from build123d import *

# Parameters (mm, degrees)
SKETCH_1_R               = 34.375
EXTRUDE_1_DEPTH          = 30
EXTRUDE_START            = -30
EXTRUDE_2_DEPTH          = 30
PATTERN_CIRCULAR_1_COUNT = 30
CUT_EXTRUDE_1_DEPTH      = 30


with BuildPart() as part:
    # 草图1 → 凸台-拉伸1 (new body)
    with BuildSketch(Plane.XY):
        Circle(SKETCH_1_R)
    extrude(amount=EXTRUDE_1_DEPTH)

    # 草图2 → 凸台-拉伸2 (add)
    with BuildSketch(Plane.XY.offset(30).offset(EXTRUDE_START)):
        with BuildLine():
            ThreePointArc((2.965504601, 39.889920813), (2.09343825, 39.94518139), (1.220372866, 39.981379292))
            ThreePointArc((1.220372866, 39.981379292), (-0.075113847, 37.287853424), (-0.712008739, 34.367625297))
            ThreePointArc((-0.712008739, 34.367625297), (1.799048496, 34.327890257), (4.300503339, 34.10493067))
            ThreePointArc((4.300503339, 34.10493067), (3.972344382, 37.075735127), (2.965504601, 39.889920813))
        make_face()
    extrude_2 = extrude(amount=EXTRUDE_2_DEPTH)

    # 阵列(圆周)1: 凸台-拉伸2 ×30 about axis
    pattern_circular_1_axis = Axis((0, 0, 0), (0, 0, 1))
    for i in range(1, PATTERN_CIRCULAR_1_COUNT):
        add(extrude_2.rotate(pattern_circular_1_axis, i * 360 / PATTERN_CIRCULAR_1_COUNT))

    # 草图3 → 切除-拉伸1 (cut)
    with BuildSketch(Plane.XY.offset(30)):
        with BuildLine():
            Line((-1.5, 14.924811557), (-1.5, 0))
            Line((-1.5, 0), (1.5, 0))
            Line((1.5, 0), (1.5, 14.924811557))
            ThreePointArc((1.5, 14.924811557), (0, 15), (-1.5, 14.924811557))
        make_face()
        with BuildLine():
            Line((1.5, 0), (-1.5, 0))
            Line((-1.5, 0), (-1.5, 14.924811557))
            ThreePointArc((-1.5, 14.924811557), (-10.062305899, -11.124297731), (15, 0))
            ThreePointArc((15, 0), (11.124297731, 10.062305899), (1.5, 14.924811557))
            Line((1.5, 14.924811557), (1.5, 0))
        make_face()
        with BuildLine():
            Line((-1.5, 17), (-1.5, 14.924811557))
            ThreePointArc((-1.5, 14.924811557), (0, 15), (1.5, 14.924811557))
            Line((1.5, 14.924811557), (1.5, 17))
            Line((1.5, 17), (-1.5, 17))
        make_face()
    extrude(amount=-CUT_EXTRUDE_1_DEPTH, mode=Mode.SUBTRACT)


solid = part.part
Could you check a few things on this model? Use its own coordinates, in mm. A direction names the side the tool comes from. Give positions to 0.01 mm unless a question says otherwise; leave off trailing zeros. Write each question's results on one line, items separated by ' | '. Start each with the question number.
Q1. I need wall thicknesses on probe 1 along X at (y, z) = (6, 15.75); probe 2 along Y at (x, z) = (10.5, 3.5); probe 3 along X at (y, z) = (24, 18). Which ranges of each line are inside material? Lowest first, please.
Q2. Which directions (+Z, -Z, +X, -X, +Y, -Y) give clear straight access to the entire face, cutting with the end or side of a thin tool? Please do faces 1 (the face through (-35.52, 11.476, 14.79)), 2 (the face through (15.1, 34.1, 14.8)), 3 (the face through (34.327, -1.814, 14.79)), 4 (the face through (1.5, 16, 15)).
Q3. I'm going to push flat-ended pins straight in: pin 1 Ø1 at (y, z) = (15.5, 12) entering from +X; pin 2 Ø1.5 at (y, z) = (-18.5, 22.5) entering from +X; pin 3 Ø6 at (x, z) = (21.5, 16) entering from -Y. Where does each tip first touch, or does it pass through?
Outcome:
1) probe 1: -39.55 to -13.75, 13.75 to 33.85 | probe 2: -34.03 to -10.71, 10.71 to 38.6 | probe 3: -27.22 to 24.61, 25.75 to 31.42
2) face 1: +Z, -Z, -X | face 2: +Z, -Z, +Y | face 3: +Z, -Z, +X | face 4: +Z, -Z
3) pin 1: x = 34.97 | pin 2: x = 32.87 | pin 3: y = -34.01
